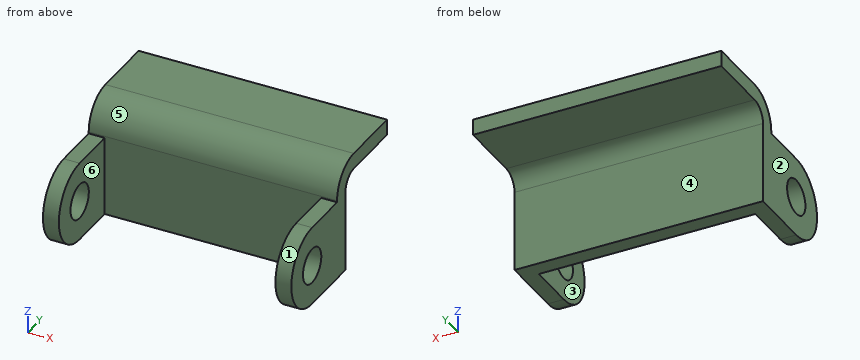
```python
from build123d import *

# Parameters (mm, degrees)
BOSS_EXTRUDE1_DEPTH = 39
SKETCH3_R           = 5.5
BOSS_EXTRUDE2_DEPTH = 5


with BuildPart() as part:
    # Sketch1 → Boss-Extrude1 (new, symmetric)
    with BuildSketch(Plane.YZ):
        with BuildLine():
            Line((-156.635856385, -79.593365073), (-176.635856385, -79.593365073))
            ThreePointArc((-176.635856385, -79.593365073), (-183.706924197, -82.522297262), (-186.635856385, -89.593365073))
            Line((-186.635856385, -89.593365073), (-186.635856385, -115.093365073))
            Line((-186.635856385, -115.093365073), (-181.635856385, -115.093365073))
            Line((-181.635856385, -115.093365073), (-181.635856385, -89.593365073))
            ThreePointArc((-181.635856385, -89.593365073), (-180.171390291, -86.057831168), (-176.635856385, -84.593365073))
            Line((-176.635856385, -84.593365073), (-156.635856385, -84.593365073))
            Line((-156.635856385, -84.593365073), (-156.635856385, -79.593365073))
        make_face()
    extrude(amount=BOSS_EXTRUDE1_DEPTH, both=True)

    # Sketch3 → Boss-Extrude2 (add)
    with BuildSketch(Plane.YZ.offset(39)):
        with BuildLine():
            Line((-181.635856385, -115.093365073), (-201.635856385, -115.093365073))
            ThreePointArc((-201.635856385, -115.093365073), (-214.13814738, -102.591074078), (-201.635856385, -90.088783083))
            Line((-201.635856385, -90.088783083), (-181.635856385, -90.088783083))
            Line((-181.635856385, -90.088783083), (-181.635856385, -115.093365073))
        make_face()
        with Locations(Location((-201.635856385, -102.591074078, 0), (0, 0, 270))):
            Circle(SKETCH3_R, mode=Mode.SUBTRACT)
    boss_extrude2 = extrude(amount=-BOSS_EXTRUDE2_DEPTH)

    # Mirror1: Boss-Extrude2 across plane
    add(boss_extrude2.mirror(Plane(origin=(0, 0, 0), x_dir=(0, 0, 1), z_dir=(1, 0, 0))))


solid = part.part
```
CAD build for the part. Positions are in the model's coordinates, mm. Face numbers are marked on the shaded views. A direction names the side the tool comes from. Give positions to 0.01 mm unless a question says otherwise; leave off trailing zeros. Loops run counter-clockwise (first coordinate to the right, second up) from the corner with the lowest first, then second, coordinate; pieces in that order, holes last. Notation, with made-up numbers: (81.5, -36.5) -> (97.5, -36.5) arc R21 ccw to (97.5, 2.5) -> close; hole circle Ø11 at (11.25, 81). An arc over 180 degrees is marked (long way). Use a Markdown table: item, result.
1. Slice it at A-A (y = -187.5). List the corners of the cut face in (x, z), plus the area to 3 significant figures.
Check result:
| item | result |
|---|---|
| outline | (-39, -115.09) -> (-34, -115.09) -> (-34, -90.09) -> (-39, -90.09) -> close; (34, -115.09) -> (39, -115.09) -> (39, -90.09) -> (34, -90.09) -> close |
| area | 250 mm^2 |
2. Flat gauge pins, fed straight in: pin 1 (12 mm diameter, centred on x = -25.5, y = -194, fed in from +Z); pin 2 (13 mm diameter, centred on x = 0, z = -97.5, fed in from -Y); pin 3 (10 mm diameter, centred on x = 6, y = -164.5, fed in from -Z); pin 4 (20.5 mm diameter, centred on x = -7.5, z = -99.5, fed in from +Y). Where does each tip first touch, or does it go through?
Check result:
| item | result |
|---|---|
| pin 1 | passes through |
| pin 2 | stops at y = -186.64 |
| pin 3 | stops at z = -84.59 |
| pin 4 | stops at y = -181.62 |
3. Slice it at B-B (y = -197). List the corners of the cut face in (x, z), plus the area to 3 significant figures.
Check result:
| item | result |
|---|---|
| outline | (-39, -115.09) -> (-34, -115.09) -> (-34, -105.55) -> (-39, -105.55) -> close; (-39, -99.63) -> (-34, -99.63) -> (-34, -90.09) -> (-39, -90.09) -> close; (34, -115.09) -> (39, -115.09) -> (39, -105.55) -> (34, -105.55) -> close; (34, -99.63) -> (39, -99.63) -> (39, -90.09) -> (34, -90.09) -> close |
| area | 191 mm^2 |
4. Slice it at D-D (x = 26.5). List the corners of the cut face in (y, z), plus the area to 3 significant figures.
Check result:
| item | result |
|---|---|
| outline | (-186.64, -115.09) -> (-181.64, -115.09) -> (-181.64, -89.59) arc R5 cw to (-176.64, -84.59) -> (-156.64, -84.59) -> (-156.64, -79.59) -> (-176.64, -79.59) arc R10 ccw to (-186.64, -89.59) -> close |
| area | 286 mm^2 |
5. Which spindle directions (+Z, -Z, +X, -X, +Y, -Y) get a long thin tool onto all of the face, cutting with end or side? Do the marked faces 4, 5 and 6. Say none if no direction does.
Check result:
| item | result |
|---|---|
| face 4 | -Z, +X, -X, +Y |
| face 5 | +Z, +X, -X, -Y |
| face 6 | +Z, -Z, -Y |
6. Wall check: L1, parallel to Y at x = -6.5, z = -91.5; L2, parallel to Z at x = 14, y = -173; L3, parallel to Z at x = 8, y = -183. Give the ranges that are in metal, low to high. Write a range as [from, to].
Check result:
| item | result |
|---|---|
| L1 | y = [-186.64, -181.64] |
| L2 | z = [-84.59, -79.59] |
| L3 | z = [-115.09, -81.88] |
7. Slice it at C-C (z = -102.5). List the corners of the cut face in (x, y).
Check result:
| item | result |
|---|---|
| outline | (-39, -214.14) -> (-34, -214.14) -> (-34, -207.14) -> (-39, -207.14) -> close; (-39, -196.14) -> (-34, -196.14) -> (-34, -186.64) -> (34, -186.64) -> (34, -196.14) -> (39, -196.14) -> (39, -181.64) -> (-39, -181.64) -> close; (34, -214.14) -> (39, -214.14) -> (39, -207.14) -> (34, -207.14) -> close |
8. Mould opens along X. For the marked faces 1, 2 and 3 say: pulls with the +X half, pulls with the -X half, needs draft (parallel to the pull), parting line crosses it, or undercut.
Check result:
| item | result |
|---|---|
| face 1 | needs draft |
| face 2 | pulls with the -X half |
| face 3 | undercut |
